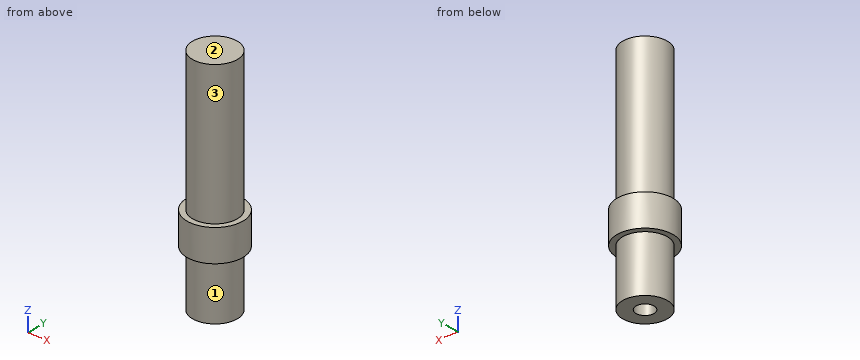
Solid Edge part; units mm, degrees
sketch "Sketch1" plane through (0, 0, 0) normal (0, 0, 1) x (1, 0, 0)
  circle A0 centre (0, 0) radius 4
extrude "Protrusion1" add sketch "Sketch1" along normal blind 10
sketch "Sketch2" plane through (0, 0, 10) normal (0, 0, 1) x (1, 0, 0)
  circle A0 centre (0, 0) radius 5
extrude "ExtrudedProtrusion_2" add sketch "Sketch2" along normal blind 5.7
sketch "Sketch3" plane through (0, 0, 15.7) normal (0, 0, 1) x (1, 0, 0)
  circle A0 centre (0, 0) radius 4
extrude "ExtrudedProtrusion_3" add sketch "Sketch3" along normal blind 25
hole "Hole_1" at (0, 0, 0) direction (0, 0, 1) diameter 3.242 depth 8
cosmetic_thread "Thread1"
properties material "Aluminum, 6061-T6"
Geometry: final body of the model. Coordinates: model frame, mm. Face numbers are marked on the shaded views. A direction names the side the tool comes from. Give positions to 0.01 mm unless a question says otherwise; leave off trailing zeros. Write each loop counter-clockwise with the first axis right and the second up, starting at its lowest first coordinate (ties: lowest second). Pieces come first, ordered by that corner, then holes. Notation, with made-up numbers: M -19,-10.5 L 0,-10.5 A22 ccw 0,0.5 Z; hole C -26,-18 d4. An arc over 180 degrees is marked long. Answer in a Markdown table with one row per item. Add a question column.
(1) Section D-D on y = -2. Return loops of the section in (x, z).
(2) Reachability of the marked faces 1, 2 and 3 from +Z, -Z, +X, -X, +Y, -Y: full face, straight path, thin tool, end or side. Return the list, or none.
(3) First-contact query: pin 1 (3 mm diameter, centred on y = -2, z = 23, fed in from +X); pin 2 (6 mm diameter, centred on x = 4, z = 29.5, fed in from +Y); pin 3 (1.9 mm diameter, centred on x = 0, y = 0, fed in from -Z); pin 4 (3 mm diameter, centred on x = 1, y = -1.5, fed in from -Z). Flat tips, straight axial feed; report the tip coordinate or a pass-through.
(4) Ray query, line 1 (Y direction, x = 0, z = 6.25); line 2 (Z direction, x = 0.75, y = 4.25); line 3 (X direction, y = -1, z = 28). Return the intervals inside material, ascending.
(5) Section C-C on z = 31. Return loops of the section in (x, y).
(6) Section A-A on y = 0. Return loops of the section in (x, z).
Result set:
| question | item | result |
|---|---|---|
| 1 | outline | M -4.58,10 L -3.46,10 L -3.46,0 L 3.46,0 L 3.46,10 L 4.58,10 L 4.58,15.7 L 3.46,15.7 L 3.46,40.7 L -3.46,40.7 L -3.46,15.7 L -4.58,15.7 Z |
| 2 | face 1 | -Z |
| 2 | face 2 | +Z, +X, -X, +Y, -Y |
| 2 | face 3 | +Z |
| 3 | pin 1 | stops at x = 3.97 |
| 3 | pin 2 | stops at y = 3.87 |
| 3 | pin 3 | stops at z = 8 |
| 3 | pin 4 | stops at z = 0 |
| 4 | line 1 | y = -4 to -1.62, 1.62 to 4 |
| 4 | line 2 | z = 10 to 15.7 |
| 4 | line 3 | x = -3.87 to 3.87 |
| 5 | outline | C 0,0 d8 |
| 6 | outline | M -5,10 L -4,10 L -4,0 L -1.62,0 L -1.62,8 L 1.62,8 L 1.62,0 L 4,0 L 4,10 L 5,10 L 5,15.7 L 4,15.7 L 4,40.7 L -4,40.7 L -4,15.7 L -5,15.7 Z |
